```python
from build123d import *

# Parameters (mm, degrees)
BOSS_EXTRUDE3_DEPTH = 40
CUT_EXTRUDE1_DEPTH  = 73.265136823
CUT_EXTRUDE2_DEPTH  = 10


with BuildPart() as part:
    # Sketch1 → Boss-Extrude3 (new body)
    with BuildSketch(Plane.XY):
        with BuildLine():
            Line((-37, -6.5), (0, -6.5))
            ThreePointArc((0, -6.5), (4.596194078, -4.596194078), (6.5, 0))
            Line((6.5, 0), (6.5, 27))
            ThreePointArc((6.5, 27), (4.596194078, 31.596194078), (0, 33.5))
            Line((0, 33.5), (-37, 33.5))
            ThreePointArc((-37, 33.5), (-41.596194078, 31.596194078), (-43.5, 27))
            Line((-43.5, 27), (-43.5, 0))
            ThreePointArc((-43.5, 0), (-41.596194078, -4.596194078), (-37, -6.5))
        make_face()
    extrude(amount=BOSS_EXTRUDE3_DEPTH)

    # Sketch3 → Cut-Extrude1 (cut, through all)
    with BuildSketch(Plane(origin=(6.5, 0, 0), x_dir=(0, 0, -1), z_dir=(1, 0, 0))):
        with BuildLine():
            Line((-27.850101272, 18.5), (-40, 18.5))
            Line((-40, 18.5), (-40, 33.5))
            Line((-40, 33.5), (-15.004868693, 33.5))
            ThreePointArc((-15.004868693, 33.5), (-17.975892442, 23.044232737), (-27.850101272, 18.5))
        make_face()
        with BuildLine():
            Line((-40, 8.5), (-40, -6.5))
            Line((-40, -6.5), (-15, -6.5))
            ThreePointArc((-15, -6.5), (-17.97102375, 3.955767263), (-27.845232579, 8.5))
            Line((-27.845232579, 8.5), (-40, 8.5))
        make_face()
    extrude(amount=-CUT_EXTRUDE1_DEPTH, mode=Mode.SUBTRACT)

    # Sketch4 → Cut-Extrude2 (cut)
    with BuildSketch(Plane(origin=(0, 18.5, 0), x_dir=(1, 0, 0), z_dir=(0, 1, 0))):
        with BuildLine():
            Line((-10.5, -40), (-26.5, -40))
            ThreePointArc((-26.5, -40), (-18.5, -32), (-10.5, -40))
        make_face()
    extrude(amount=-CUT_EXTRUDE2_DEPTH, mode=Mode.SUBTRACT)


solid = part.part
```
The model under review builds one solid part; all positions refer to its coordinate system, in mm. A direction names the side the tool comes from. Coordinates: 2 decimals unless noted, no trailing zeros. Write each loop counter-clockwise with the first axis right and the second up, starting at its lowest first coordinate (ties: lowest second). Pieces come first, ordered by that corner, then holes. Notation, with made-up numbers: (68.25, 7) - (82.25, 7) arc R24 ccw to (82.25, 25) - close; hole circle Ø6 at (-34, 44.5). An arc over 180 degrees is marked (long way). Answer in a Markdown table with one row per item. Add a question column.
Q1. Clearance check with flat-ended pins moving along their axes: pin 1 (6 mm diameter, centred on x = -7, z = 32, fed in from +Y); pin 2 (2 mm diameter, centred on x = -18.5, y = 16.5, fed in from +Z); pin 3 (3.5 mm diameter, centred on x = -24, z = 36, fed in from -Y). State where each tip first meets the part, or that it passes through.
Q2. Consider section B-B on x = -28. Give the boundary of the cut face in (y, z), then the cut area to 3 significant figures.
Q3. Consider section A-A on y = 17. Give the boundary of the cut face in (x, z).
Q4. Draft analysis for pull direction Y (two halves, no side actions). For faces 4 (the face through (-2, 14, 40)), 5 (the face through (-41.646, -4.545, 7.715)), 6 (the face through (-18.15, 23.164, 17.874)), state which applies: +Y half, -Y half, draft (parallel to the pull), parting line (faces both ways), or undercut.
Q5. Consider section D-D on z = 19. Give the boundary of the cut face in (x, y), then the cut area to 3 significant figures.
Q6. To check wall thickness, follow line 1 along Z through (x, y) = (-29.5, 29.5); line 2 along Z through (x, y) = (1.5, -4.5); line 3 along Y through (x, z) = (-17.5, 29.5). State the ranges of each line that lie inside material, in increasing order. Write a range as from..to.
Q7. For faces 1 (the face through (-18.15, 3.836, 17.87)), 2 (the face through (-18, 8.5, 31)), 3 (the face through (-18, 18.5, 31)), list the 3-axis set-ups (+Z, -Z, +X, -X, +Y, -Y) from which the entire face can be reached by the end or side of a thin tool; tool diameter is ignored.
Q8. Consider section C-C on z = 5. Give the boundary of the cut face in (x, y), then the cut area to 3 significant figures.
Answers below:
| question | item | result |
|---|---|---|
| 1 | pin 1 | y = 18.5 |
| 1 | pin 2 | z = 32.06 |
| 1 | pin 3 | y = 8.5 |
| 2 | outline | (-6.5, 0) - (33.5, 0) - (33.5, 15) arc R13 cw to (18.5, 27.85) - (18.5, 40) - (8.5, 40) - (8.5, 27.85) arc R13 cw to (-6.5, 15) - close |
| 2 | area | 918 mm² |
| 3 | outline | (-43.5, 0) - (6.5, 0) - (6.5, 40) - (-10.5, 40) arc R8 cw to (-26.5, 40) - (-43.5, 40) - close |
| 4 | face 4 | draft |
| 4 | face 5 | -Y half |
| 4 | face 6 | undercut |
| 5 | outline | (-43.5, 5.03) - (6.5, 5.03) - (6.5, 21.98) - (-43.5, 21.98) - close |
| 5 | area | 848 mm² |
| 6 | line 1 | 0..15 |
| 6 | line 2 | 0..14.85 |
| 6 | line 3 | 8.5..18.5 |
| 7 | face 1 | +Z, +X, -X |
| 7 | face 2 | +Z, +X, -X, -Y |
| 7 | face 3 | +Z, +X, -X, +Y |
| 8 | outline | (-43.5, 0) arc R6.5 ccw to (-37, -6.5) - (0, -6.5) arc R6.5 ccw to (6.5, 0) - (6.5, 27) arc R6.5 ccw to (0, 33.5) - (-37, 33.5) arc R6.5 ccw to (-43.5, 27) - close |
| 8 | area | 1,960 mm² |
